Autodesk Inventor part; units mm, degrees
ref_plane "YZ Plane" through (0, 0, 0) normal (1, 0, 0) x (0, 1, 0)
ref_plane "XY Plane" through (0, 0, 0) normal (0, 0, 1) x (1, 0, 0)
sketch "Sketch1" plane through (0, 0, 0) normal (0, 1, 0) x (-1, 0, 0)
  line L0 (0, -18.13) -> (0, 18.13) construction
  line L1 (-3.6, 0) -> (0.6, 0) construction
  line L2 (0, 12.95) -> (-3, 12.95)
  line L3 (-3, 12.95) -> (-3, -12.95)
  line L4 (-3, -12.95) -> (0, -12.95)
  line L5 (0, 12.95) -> (0, -12.95)
  point P0 (0, 0)
  dimension "d0" = 3
  dimension "d1" = 25.9
revolve "Revolution1" add sketch "Sketch1" angle 360 about axis through (0, 0, 12.95) along (0, 0, -1)
sketch "Sketch2" plane through (0, 0, 0) normal (0, 1, 0) x (-1, 0, 0)
  line L0 (0, -18.2) -> (0, 18.2) construction
  line L1 (-4.2, 0) -> (4.2, 0) construction
  line L2 (-3, 12.95) -> (-3, 12.95)
  line L3 (-3, 4.25) -> (-2.85, 4.25)
  line L4 (-2.85, 4.25) -> (-2.85, 5.05)
  line L5 (-2.85, 5.05) -> (-3, 5.05)
  line L6 (-3, 5.05) -> (-3, 4.25)
  line L7 (-3, 4.25) -> (-3, 5.05)
  line L8 (-3, -12.95) -> (-3, 12.95)
  line L9 (3, 12.95) -> (-3, 12.95)
  line L10 (-3, -1.55) -> (-2.85, -1.55)
  line L11 (-2.85, -1.55) -> (-2.85, -2.35)
  line L12 (-2.85, -2.35) -> (-3, -2.35)
  line L13 (-3, -2.35) -> (-3, -1.55)
  line L14 (-3, -3.35) -> (-2.85, -3.35)
  line L15 (-2.85, -3.35) -> (-2.85, -4.15)
  line L16 (-2.85, -4.15) -> (-3, -4.15)
  line L17 (-3, -4.15) -> (-3, -3.35)
  line L18 (-3, -11.15) -> (-2.85, -11.15)
  line L19 (-2.85, -11.15) -> (-2.85, -11.95)
  line L20 (-2.85, -11.95) -> (-3, -11.95)
  line L21 (-3, -11.95) -> (-3, -11.15)
  line L22 (3, -12.95) -> (-3, -12.95)
  point P0 (-3, -2.35)
  point P1 (-3, -4.15)
  point P2 (-3, -11.95)
  dimension "d34" = 0.8
  dimension "d35" = 2.85
  dimension "d57" = 5.8
  dimension "d58" = 7
  dimension "d59" = 1
  dimension "d63" = 1
revolve "Revolution2" cut sketch "Sketch2" angle 360 about axis through (0, 0, 0) along (0, 0, 1)
ref_plane "Work Plane2" through (0, 3, 0) normal (0, 1, 0) x (-1, 0, 0)
sketch "Sketch4" plane through (0, 3, 0) normal (0, 1, 0) x (-1, 0, 0)
  line L0 (0, -26.0074) -> (0, 32.7926) construction
  line L1 (1, -9.725) -> (1, -5.575)
  line L2 (-1, -5.575) -> (-1, -9.725)
  arc A0 (-1, -9.725) -> (1, -9.725) centre (0, -9.725) ccw
  arc A1 (1, -5.575) -> (-1, -5.575) centre (0, -5.575) ccw
  line L3 (3, -12.95) -> (-3, -12.95)
  line L4 (-1, -7.65) -> (1, -7.65) construction
  line L5 (-3, -4.15) -> (3, -4.15) construction
  line L6 (3, -11.15) -> (-3, -11.15) construction
  line L7 (0, -17.6074) -> (0, 24.3926) construction
  line L8 (1, 7.05) -> (1, 11.2)
  line L9 (-1, 11.2) -> (-1, 7.05)
  arc A2 (-1, 7.05) -> (1, 7.05) centre (0, 7.05) ccw
  arc A3 (1, 11.2) -> (-1, 11.2) centre (0, 11.2) ccw
  line L10 (3, 12.95) -> (-3, 12.95)
  point P0 (0, 0)
  point P1 (1, 1)
  point P2 (0, 24.3926)
  dimension "d49" = 6.15
  dimension "d50" = 1
  dimension "d60" = 3.5
  dimension "d61" = 3.5
  dimension "d64" = 6.15
  dimension "d65" = 1
  dimension "d66" = 1.75
extrude "Extrusion2" cut sketch "Sketch4" against normal blind 1
chamfer "Chamfer3" distance 0.5 angle 45 2 edges at (-3, 0, -12.95) (-3, 0, 12.95)
equation "\"module\" = 1"
equation "\"pressure_ang\" = 30deg"
equation "\"pitch\" = 3.1416 * module"
equation "\"addendum\" = 0.45 * module"
equation "\"dedendum\" = 0.65 * module"
equation "\"tooth_depth\" = addendum + dedendum"
equation "\"addendum_mod_shaft\" = 0.45 * module"
equation "\"root_fillet_r\" = 0.16 * module"
equation "\"addendum_mod_hub\" = -addendum_mod_shaft"
equation "\"nom_space_t_hub\" = nom_tooth_t_shaft"
properties part number "Shaft_stage_input" material "Steel"
CAD build for the part. Positions are in the model's coordinates, mm. A direction names the side the tool comes from. Give positions to 0.01 mm unless a question says otherwise; leave off trailing zeros. Loops run counter-clockwise (first coordinate to the right, second up) from the corner with the lowest first, then second, coordinate; pieces in that order, holes last. Notation, with made-up numbers: M -39,73 L 0,73 A17 cw 0,77 Z; hole C 22.5,-37.75 d2. An arc over 180 degrees is marked long. Write each question's results on one line, items separated by ' | '.
Q1. Flat gauge pins, fed straight in: P1, Ø0.9, axis at y = 2.5, z = 10, coming from the -X side; P2, Ø0.7, axis at y = 2.5, z = -8.5, coming from the -X side; P3, Ø1.5, axis at y = -1.5, z = -0.5, coming from the +X side; P4, Ø1, axis at y = 0.5, z = 0.5, coming from the +X side. Where does each tip first touch, or does it go through?
Geometry check:
P1: stops at x = -2.19 | P2: stops at x = -2.09 | P3: stops at x = 2.9 | P4: stops at x = 3
Q2. Band-saw the part on A-A on z = -7.75. Write the cut outline in (x, y).
Geometry check:
outline: M -1,2 L -1,2.83 A3 ccw long 1,2.83 L 1,2 Z
Q3. Mould opens along X. For faces 4 (the face through (0, 0, 12.95)), 5 (the face through (-2.262, -1.734, 4.656)), 6 (the face through (-1, 2.4, 9.1)) say: pulls with the +X half, pulls with the -X half, needs draft (parallel to the pull), parting line crosses it, or undercut.
Geometry check:
face 4: needs draft | face 5: parting line crosses it | face 6: undercut
Q4. Probe probe 1 along Y at (x, z) = (-1.75, -9.5); probe 2 along X at (y, z) = (-0.75, -0.25). List the from-to ranges inside material, lowest first.
Geometry check:
probe 1: y = -2.44 to 2.44 | probe 2: x = -2.9 to 2.9
Q5. Band-saw the part on C-C on z = -10.5. Write the cut outline in (x, y), and give its area (3 significant figures).
Geometry check:
outline: M -0.63,2 L -0.63,2.93 A3 ccw long 0.63,2.93 L 0.63,2 Z | area: 27.0 mm²
Q6. Which spindle directions (+Z, -Z, +X, -X, +Y, -Y) get a long thin tool onto all of the face, cutting with end or side? Do faces 1 (the face through (-2.262, 1.734, -1.956)), 2 (the face through (0, 2.5, 12.2)), 3 (the face through (-3, 0, 1)). Say none if no direction does.
Geometry check:
face 1: none | face 2: +Y | face 3: +Z, -Z
Q7. Band-saw the part on B-B on z = 3. Write the cut outline in (x, y), and give its area (3 significant figures).
Geometry check:
outline: C 0,0 d6 | area: 28.3 mm²
